```python
from build123d import *

# Parameters (mm, degrees)
BOSS_EXTRUDE1_DEPTH = 3
SKETCH2_R           = 1
BOSS_EXTRUDE2_DEPTH = 3
SKETCH3_R           = 1
BOSS_EXTRUDE3_DEPTH = 3


with BuildPart() as part:
    # Sketch1 → Boss-Extrude1 (new body)
    with BuildSketch(Plane.XY):
        with BuildLine():
            ThreePointArc((-8.738694844, 5.390391994), (-9.738694844, 4.390391994), (-8.738694844, 3.390391994))
            Line((-8.738694844, 3.390391994), (-8.470745652, 3.390391994))
            ThreePointArc((-8.470745652, 3.390391994), (-4.738694844, 4.390391994), (-8.470745652, 5.390391994))
            Line((-8.470745652, 5.390391994), (-8.738694844, 5.390391994))
        make_face()
    extrude(amount=BOSS_EXTRUDE1_DEPTH)

    # Sketch2 → Boss-Extrude2 (add)
    with BuildSketch(Plane.XY.offset(3)):
        with Locations((-8.738694844, 4.390391994)):
            Circle(SKETCH2_R)
    extrude(amount=BOSS_EXTRUDE2_DEPTH)

    # Sketch3 → Boss-Extrude3 (add)
    with BuildSketch(Plane(origin=(0, 0, 0), x_dir=(-1, 0, 0), z_dir=(0, 0, -1))):
        with Locations((6.738694844, 4.390391994)):
            Circle(SKETCH3_R)
    extrude(amount=BOSS_EXTRUDE3_DEPTH)


solid = part.part
```
Source: CAD feature listing. Evaluate the final solid. Frame: model axes, mm. A direction names the side the tool comes from. Coordinates: 2 decimals unless noted, no trailing zeros. Write each loop counter-clockwise with the first axis right and the second up, starting at its lowest first coordinate (ties: lowest second). Pieces come first, ordered by that corner, then holes. Notation, with made-up numbers: M 89.5,-33.5 L 140.5,-33.5 A29 ccw 140.5,-0.5 Z; hole C 75,7.25 d7. An arc over 180 degrees is marked long. Answer as a JSON object with one key per item and string values.
1. Access query for faces 1 (the flat face through (-9, 4, 6)), 2 (the cylindrical face through (-6.002, 5.066, -1.479)), 3 (the cylindrical face through (-9.738, 4.434, 3.625)). Directions: +Z, -Z, +X, -X, +Y, -Y. A direction counts if a zero-diameter tool reaches every point of the face in a straight line with its end or side. Return the directions, or none.
Evaluation:
{"face 1": "+Z, +X, -X, +Y, -Y", "face 2": "-Z", "face 3": "+Z"}
2. Cut plane A-A on y = 4.05. Output: boundary loops of the cut face in (x, z).
Evaluation:
{"outline": "M -9.68,0 L -7.68,0 L -7.68,-3 L -5.8,-3 L -5.8,0 L -4.77,0 L -4.77,3 L -7.8,3 L -7.8,6 L -9.68,6 Z"}
3. Ray query, L1, parallel to Z at x = -6.7, y = 3; L2, parallel to Z at x = -6, y = 4.9; L3, parallel to X at y = 4.4, z = -2.25. Return the intervals inside material, ascending.
Evaluation:
{"L1": "0 to 3", "L2": "-3 to 3", "L3": "-7.74 to -5.74"}
4. Cut plane D-D on y = 4.75. Output: boundary loops of the cut face in (x, z).
Evaluation:
{"outline": "M -9.67,0 L -7.67,0 L -7.67,-3 L -5.81,-3 L -5.81,0 L -4.77,0 L -4.77,3 L -7.81,3 L -7.81,6 L -9.67,6 Z"}
5. Contact query for flat-ended pins moving along their axis: P1, Ø1.2, axis at x = -7, y = 4, coming from the +Z side; P2, Ø1, axis at y = 3.5, z = 1.5, coming from the +X side; P3, Ø1.5, axis at x = -5.5, z = 3.5, coming from the -Y side. Output: stop coordinate, or through.
Evaluation:
{"P1": "z = 3", "P2": "x = -4.78", "P3": "y = 2.51"}
6. Cut plane C-C on z = 0.5. Output: boundary loops of the cut face in (x, y).
Evaluation:
{"outline": "M -8.74,3.39 L -8.47,3.39 A2 ccw long -8.47,5.39 L -8.74,5.39 A1 ccw Z"}
7. Cut plane B-B on x = -7.4. Output: boundary loops of the cut face in (y, z).
Evaluation:
{"outline": "M 2.5,0 L 3.64,0 L 3.64,-3 L 5.14,-3 L 5.14,0 L 6.28,0 L 6.28,3 L 2.5,3 Z"}
